Could you check a few things on this model? Use its own coordinates, in mm. Round coordinates to 2 decimals unless told otherwise and drop trailing zeros. Order: outer loops, then holes, each group sorted by start corner. A loop starts at its lowest first (then second) coordinate and runs counter-clockwise, first axis right, second up. Notation, with made-up numbers: (81, 36.25) - (113, 36.25) arc R24 ccw to (113, 65.25) - close; hole circle Ø9 at (46, 70.25). An arc over 180 degrees is marked (long way). Use one line per item in the form item = value.
from build123d import *

# Parameters (mm, degrees)
MODEL_R         = 4.5
MODEL_W         = 10
MODEL_H         = 4.4
MODEL_H_2       = 2.2
EXTRUDE_1_DEPTH = 1


with BuildPart() as part:
    # Model → 凸台-拉伸1 (new body)
    with BuildSketch(Plane.XY):
        Polygon((4.031012873, 85.725728146), (53.031012873, 85.725728146), (53.031012873, 63.624082732), (51.031012873, 63.624082732), (51.031012873, 33.624082732), (53.031012873, 33.624082732), (53.031012873, 3.624082732), (34.281012873, 3.624082732), (34.281012873, 18.724082732), (28.531012873, 18.724082732), (22.781012873, 18.724082732), (22.781012873, 3.624082732), (4.031012873, 3.624082732), (4.031012873, 33.624082732), (6.031012873, 33.624082732), (6.031012873, 63.624082732), (4.031012873, 63.624082732), align=None)
        with Locations((28.531012873, 43.724082732)):
            Circle(MODEL_R, mode=Mode.SUBTRACT)
        with Locations((36.031012873, 78.525728146)):
            Rectangle(MODEL_W, MODEL_H, mode=Mode.SUBTRACT)
        with Locations((21.031012873, 78.525728146)):
            Rectangle(MODEL_W, MODEL_H, mode=Mode.SUBTRACT)
        with Locations((21.031012873, 28.897146128)):
            Rectangle(MODEL_W, MODEL_H_2, mode=Mode.SUBTRACT)
        with Locations((36.031012873, 28.897146128)):
            Rectangle(MODEL_W, MODEL_H_2, mode=Mode.SUBTRACT)
    extrude(amount=EXTRUDE_1_DEPTH)


solid = part.part
Item 1: Imagine slicing it at C-C on z = 0.25. State how many separate pieces and enclosed holes the cut face has, plus the area to 3 significant figures.
Found:
separate_pieces = 1
enclosed_holes = 5
area = 3,530 mm2
Item 2: Will this pin go through, and if not, where does the flat tip stop? P1, Ø0.5, axis at x = 30, z = 0.5, coming from the -Y side.
Found:
P1 = 18.72
Item 3: Imagine slicing it at A-A on y = 12. Please give me the cut outline in (x, z), plus the area to 3 significant figures.
Found:
outline = (4.03, 0) - (22.78, 0) - (22.78, 1) - (4.03, 1) - close; (34.28, 0) - (53.03, 0) - (53.03, 1) - (34.28, 1) - close
area = 37.5 mm2
Item 4: Imagine slicing it at D-D on x = 29. Please give me the cut outline in (y, z), plus the area to 3 significant figures.
Found:
outline = (18.72, 0) - (39.25, 0) - (39.25, 1) - (18.72, 1) - close; (48.2, 0) - (85.73, 0) - (85.73, 1) - (48.2, 1) - close
area = 58.1 mm2
Item 5: Imagine slicing it at B-B on x = 20. Please give me the cut outline in (y, z), plus the area to 3 significant figures.
Found:
outline = (3.62, 0) - (27.8, 0) - (27.8, 1) - (3.62, 1) - close; (30, 0) - (76.33, 0) - (76.33, 1) - (30, 1) - close; (80.73, 0) - (85.73, 0) - (85.73, 1) - (80.73, 1) - close
area = 75.5 mm2
Item 6: I need wall thicknesses on L1, parallel to Y at x = 38, z = 0.55; L2, parallel to Y at x = 34, z = 0.5; L3, parallel to X at y = 9.5, z = 0.95. Which ranges of each line are inside material? Lowest first, please.
Found:
L1 = 3.62 to 27.8, 30 to 76.33, 80.73 to 85.73
L2 = 18.72 to 27.8, 30 to 76.33, 80.73 to 85.73
L3 = 4.03 to 22.78, 34.28 to 53.03
